from build123d import *

# Parameters (mm, degrees)
SKETCH_1_W      = 44
SKETCH_1_H      = 24
EXTRUDE_1_DEPTH = 20
EXTRUDE_2_DEPTH = 3


with BuildPart() as part:
    # 草图1 → 凸台-拉伸1 (new body)
    with BuildSketch(Plane.XY):
        Rectangle(SKETCH_1_W, SKETCH_1_H)
    extrude(amount=EXTRUDE_1_DEPTH)

    # 草图2 → 凸台-拉伸2 (add)
    with BuildSketch(Plane(origin=(0, 0, 0), x_dir=(-1, 0, 0), z_dir=(0, 0, -1))):
        with BuildLine():
            Line((22, 4.523639819), (22, -1e-08))
            ThreePointArc((22, -1e-08), (22.585786434, 1.414213559), (24, 2))
            Line((24, 2), (29, 2))
            Line((29, 2), (27.809223998, 3.190776002))
            Line((27.809223998, 3.190776002), (22, 4.523639819))
        make_face()
        with BuildLine():
            Line((22, -4.523639819), (27.809223998, -3.190776002))
            Line((27.809223998, -3.190776002), (29, -2))
            Line((29, -2), (24, -2))
            ThreePointArc((24, -2), (22.585786441, -1.414213566), (22, -1e-08))
            Line((22, -1e-08), (22, -4.523639819))
        make_face()
        with BuildLine():
            Line((-27.809223998, 3.190776002), (-29, 2))
            Line((-29, 2), (-24, 2))
            ThreePointArc((-24, 2), (-22.585786447, 1.414213572), (-22, 2.8e-08))
            Line((-22, 2.8e-08), (-22, 4.523639819))
            Line((-22, 4.523639819), (-27.809223998, 3.190776002))
        make_face()
        with BuildLine():
            Line((-22, -4.523639819), (-22, 2.8e-08))
            ThreePointArc((-22, 2.8e-08), (-22.585786428, -1.414213553), (-24, -2))
            Line((-24, -2), (-29, -2))
            Line((-29, -2), (-27.809223998, -3.190776002))
            Line((-27.809223998, -3.190776002), (-22, -4.523639819))
        make_face()
    extrude(amount=-EXTRUDE_2_DEPTH)


solid = part.part
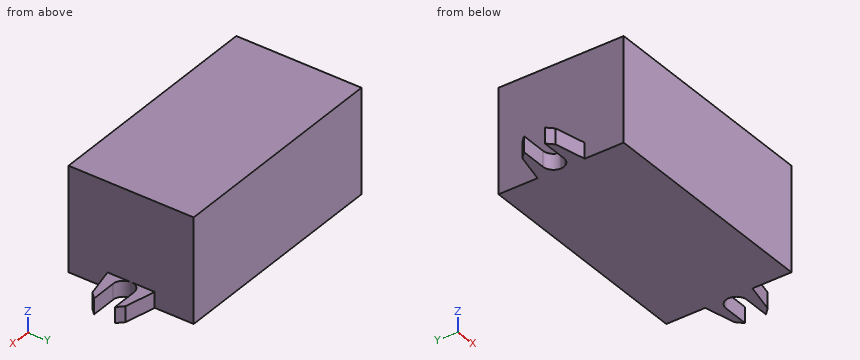
The listing builds one solid part. Answer for the finished solid, in the listing's coordinates (mm). Give positions to 0.01 mm unless a question says otherwise; leave off trailing zeros. Write each loop counter-clockwise with the first axis right and the second up, starting at its lowest first coordinate (ties: lowest second). Pieces come first, ordered by that corner, then holes.
1) Section B-B (y = 0.75) is taken. Write down the section's boundary in (x, z).
2) Given P1, Ø5, axis at x = 25, y = 1, coming from the +Z side; P2, Ø3.5, axis at x = 25.5, z = 1, coming from the -Y side; P3, Ø1.5, axis at x = -27.5, z = 2, coming from the -Y side, each flat-ended and moving along its own axis, determine where each tip first touches the part or whether it passes through.
3) Section C-C (y = -5.25) is taken. Write down the section's boundary in (x, z), and give its area (3 significant figures).
4) Section A-A (z = 1) is taken. Write down the section's boundary in (x, y).
5) Section D-D (z = 13.5) is taken. Write down the section's boundary in (x, y), and give its area (3 significant figures).
6) Find the intervals of material crossed by L1, parallel to Z at x = 26, y = -2.25; L2, parallel to X at y = 3.5, z = 6.5; L3, parallel to Y at x = -25, z = 1.5, in increasing order.
Response:
1. outline: (-22.15, 0) - (22.15, 0) - (22.15, 3) - (22, 3) - (22, 20) - (-22, 20) - (-22, 3) - (-22.15, 3) - close
2. P1: stops at z = 3
2. P2: stops at y = -4.12
2. P3: stops at y = -3.43
3. outline: (-22, 0) - (22, 0) - (22, 20) - (-22, 20) - close
3. area: 880 mm2
4. outline: (-29, -2) - (-27.81, -3.19) - (-22, -4.52) - (-22, -12) - (22, -12) - (22, -4.52) - (27.81, -3.19) - (29, -2) - (24, -2) arc R2 cw to (24, 2) - (29, 2) - (27.81, 3.19) - (22, 4.52) - (22, 12) - (-22, 12) - (-22, 4.52) - (-27.81, 3.19) - (-29, 2) - (-24, 2) arc R2 cw to (-24, -2) - close
5. outline: (-22, -12) - (22, -12) - (22, 12) - (-22, 12) - close
5. area: 1,060 mm2
6. L1: z = 0 to 3
6. L2: x = -22 to 22
6. L3: y = -3.84 to -2, 2 to 3.84
